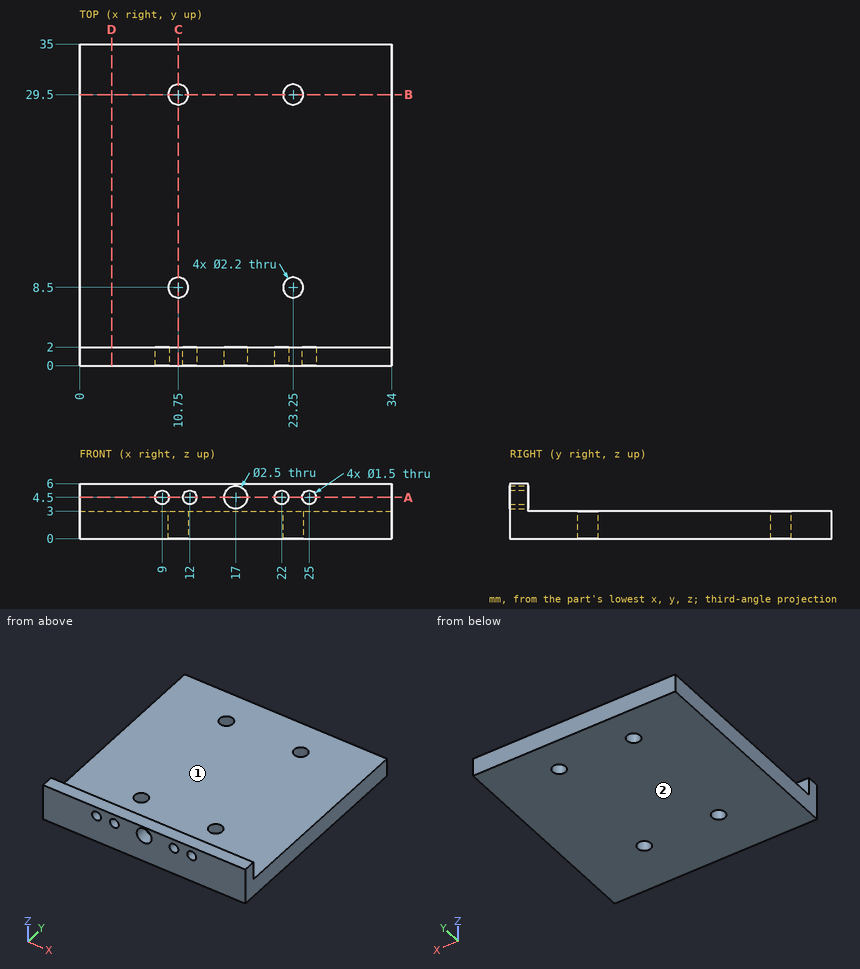
Design review of the part shown in the three views and the two pictorial views. Dimensions are in mm from the part's minimum x, y and z. A direction names the side the tool comes from. Round coordinates to 2 decimals unless told otherwise and drop trailing zeros. Loops run counter-clockwise (first coordinate to the right, second up) from the corner with the lowest first, then second, coordinate; pieces in that order, holes last.
1) Wall thickness on line 1 along Y through (x, z) = (23.25, 2.15); line 2 along X through (y, z) = (1.25, 4.5); line 3 along Y through (x, z) = (22.5, 1.15): over which ranges is each line inside the solid? List them lowest first.
Values follow:
line 1: y = 0 to 7.4, 9.6 to 28.4, 30.6 to 35
line 2: x = 0 to 8.25, 9.75 to 11.25, 12.75 to 15.75, 18.25 to 21.25, 22.75 to 24.25, 25.75 to 34
line 3: y = 0 to 7.7, 9.3 to 28.7, 30.3 to 35
2) Consider section B-B on y = 29.5. State the section outline as (x, z) points, then the cut area to 3 significant figures.
Values follow:
outline: (0, 0) - (9.65, 0) - (9.65, 3) - (0, 3) - close; (11.85, 0) - (22.15, 0) - (22.15, 3) - (11.85, 3) - close; (24.35, 0) - (34, 0) - (34, 3) - (24.35, 3) - close
area: 88.8 mm2
3) Consider section A-A on z = 4.5. State the section outline as (x, y) points, then the cut area to 3 significant figures.
Values follow:
outline: (0, 0) - (8.25, 0) - (8.25, 2) - (0, 2) - close; (9.75, 0) - (11.25, 0) - (11.25, 2) - (9.75, 2) - close; (12.75, 0) - (15.75, 0) - (15.75, 2) - (12.75, 2) - close; (18.25, 0) - (21.25, 0) - (21.25, 2) - (18.25, 2) - close; (22.75, 0) - (24.25, 0) - (24.25, 2) - (22.75, 2) - close; (25.75, 0) - (34, 0) - (34, 2) - (25.75, 2) - close
area: 51.0 mm2
4) Consider section C-C on x = 10.75. State the section outline as (y, z) points.
Values follow:
outline: (0, 0) - (7.4, 0) - (7.4, 3) - (2, 3) - (2, 6) - (0, 6) - close; (9.6, 0) - (28.4, 0) - (28.4, 3) - (9.6, 3) - close; (30.6, 0) - (35, 0) - (35, 3) - (30.6, 3) - close
5) Tool access review of the marked faces 1 and 2: name each direction out of +Z, -Z, +X, -X, +Y, -Y from which nothing blocks a thin tool from reaching the whole face with its end or side.
Values follow:
face 1: +Z, +X, -X, +Y
face 2: -Z, +X, -X, +Y, -Y
6) Consider section D-D on x = 3.5. State the section outline as (y, z) points.
Values follow:
outline: (0, 0) - (35, 0) - (35, 3) - (2, 3) - (2, 6) - (0, 6) - close
7) Clearance check with flat-ended pins moving along their axes: P1, Ø2.5, axis at x = 22.5, z = 5, coming from the +Y side; P2, Ø3, axis at x = 10.75, y = 8.5, coming from the +Z side. State where each tip first meets the part, or that it passes through.
Values follow:
P1: stops at y = 2
P2: stops at z = 3
